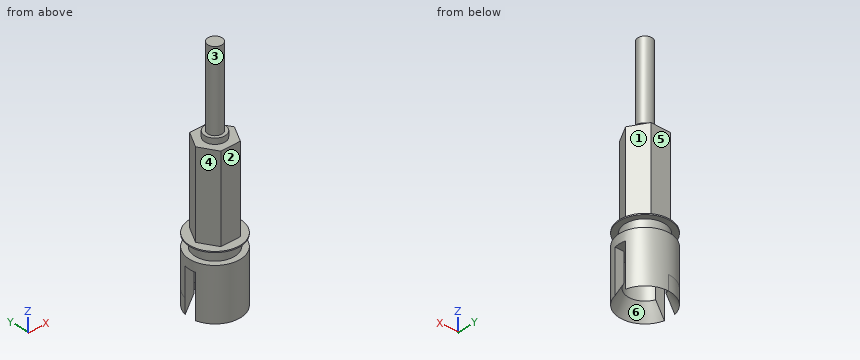
Autodesk Inventor part; units mm, degrees
ref_plane "YZ Plane" through (0, 0, 0) normal (1, 0, 0) x (0, 1, 0)
ref_plane "XZ Plane" through (0, 0, 0) normal (0, 1, 0) x (-1, 0, 0)
ref_plane "XY Plane" through (0, 0, 0) normal (0, 0, 1) x (1, 0, 0)
sketch "Sketch1" plane through (0, 0, 0) normal (0, 0, 1) x (1, 0, 0)
  line L0 (2.1997, -3.81) -> (-2.1997, -3.81)
  line L1 (-2.1997, -3.81) -> (-4.3994, 0)
  line L2 (-4.3994, 0) -> (-2.1997, 3.81)
  line L3 (-2.1997, 3.81) -> (2.1997, 3.81)
  line L4 (2.1997, 3.81) -> (4.3994, 0)
  line L5 (4.3994, 0) -> (2.1997, -3.81)
  point P0 (0, 0)
  point P1 (0, 0)
  dimension "d0" = 7.62
extrude "Extrusion1" add sketch "Sketch1" along normal blind 19.05
sketch "Sketch2" plane through (0, 0, 19.05) normal (0, 0, 1) x (1, 0, 0)
  circle A0 centre (0, 0) radius 2.286
  dimension "d3" = 4.572
extrude "Extrusion2" add sketch "Sketch2" along normal blind 1.27
sketch "Sketch3" plane through (0, 0, 20.32) normal (0, 0, 1) x (1, 0, 0)
  circle A0 centre (0, 0) radius 2.286
  circle A1 centre (0, 0) radius 1.5875
  dimension "d6" = 3.175
extrude "Extrusion3" add sketch "Sketch3" along normal blind 17.78 contours A1
thread "Thread1"
sketch "Sketch4" plane through (0, 0, 0) normal (0, 0, -1) x (-1, 0, 0)
  circle A0 centre (0, 0) radius 5.715
  dimension "d11" = 11.43
extrude "Extrusion4" add sketch "Sketch4" along normal blind 0.254
sketch "Sketch5" plane through (0, 0, -0.254) normal (0, 0, -1) x (-1, 0, 0)
  circle A0 centre (0, 0) radius 5.715
  circle A1 centre (0, 0) radius 4.445
  dimension "d14" = 8.89
extrude "Extrusion5" add sketch "Sketch5" along normal blind 2.54 contours A1
sketch "Sketch6" plane through (0, 0, -2.794) normal (0, 0, -1) x (-1, 0, 0)
  circle A0 centre (0, 0) radius 4.445
  circle A1 centre (0, 0) radius 5.715
  dimension "d17" = 11.43
extrude "Extrusion6" add sketch "Sketch6" along normal blind 2.032 contours A0 | A1
sketch "Sketch7" plane through (0, 0, -4.826) normal (0, 0, -1) x (-1, 0, 0)
  circle A0 centre (0, 0) radius 5.715
  circle A1 centre (0, 0) radius 5.715
  line L0 (0, 6.5237) -> (0, -6.5237) construction
  arc A2 (-3.5921, -1.27) -> (3.5921, -1.27) centre (0, 0) ccw
  arc A3 (3.5921, 1.27) -> (-3.5921, 1.27) centre (0, 0) ccw
  arc A4 (-5.5721, -1.27) -> (5.5721, -1.27) centre (0, 0) ccw
  arc A5 (5.5721, 1.27) -> (-5.5721, 1.27) centre (0, 0) ccw
  arc A6 (-3.5921, 1.27) -> (-3.5921, -1.27) centre (0, 0) ccw
  arc A7 (-5.5721, 1.27) -> (-5.5721, -1.27) centre (0, 0) ccw
  arc A8 (3.5921, -1.27) -> (3.5921, 1.27) centre (0, 0) ccw
  arc A9 (5.5721, -1.27) -> (5.5721, 1.27) centre (0, 0) ccw
  point P0 (-5.715, 1.27)
  point P1 (-5.715, -1.27)
  point P2 (5.715, 1.27)
  point P3 (5.715, -1.27)
extrude "Extrusion8" add sketch "Sketch7" along normal blind 6.35
sketch "Sketch13" plane through (0, 0, 0) normal (1, 0, 0) x (0, 1, 0)
  line L0 (2.286, 20.32) -> (2.286, 19.05)
  line L1 (2.286, 19.05) -> (3.81, 19.05)
  line L2 (3.81, 19.05) -> (3.81, 0)
  line L3 (3.81, 0) -> (5.715, 0)
  line L4 (5.715, 0) -> (5.715, -0.254)
  line L5 (5.715, -0.254) -> (4.445, -0.254)
  line L6 (4.445, -0.254) -> (4.445, -2.794)
  line L7 (4.445, -2.794) -> (5.715, -2.794)
  line L8 (5.715, -2.794) -> (5.715, -11.176)
  line L9 (5.715, -11.176) -> (3.81, -11.176)
  line L10 (3.81, -11.176) -> (3.81, -4.826)
  line L11 (3.81, -4.826) -> (-3.81, -4.826)
  line L12 (-3.81, -4.826) -> (-3.81, -11.176)
  line L13 (-3.81, -11.176) -> (-5.715, -11.176)
  line L14 (-5.715, -11.176) -> (-5.715, -2.794)
  line L15 (-5.715, -2.794) -> (-4.445, -2.794)
  line L16 (-4.445, -2.794) -> (-4.445, -0.254)
  line L17 (-4.445, -0.254) -> (-5.715, -0.254)
  line L18 (-5.715, -0.254) -> (-5.715, 0)
  line L19 (-5.715, 0) -> (-3.81, 0)
  line L20 (-3.81, 0) -> (-3.81, 19.05)
  line L21 (-3.81, 19.05) -> (-2.286, 19.05)
  line L22 (-2.286, 19.05) -> (-2.286, 20.32)
  line L23 (-2.286, 20.32) -> (-1.5875, 20.32)
  line L24 (-1.5875, 20.32) -> (-1.5875, 38.1)
  line L25 (-1.5875, 38.1) -> (1.5875, 38.1)
  line L26 (1.5875, 38.1) -> (1.5875, 20.32)
  line L27 (1.5875, 20.32) -> (2.286, 20.32)
  line L28 (5.715, -11.176) -> (5.715, -14.4756)
  line L29 (5.715, -14.4756) -> (3.81, -11.176)
  line L30 (3.81, -11.176) -> (5.715, -11.176)
  line L31 (0, -24.9907) -> (0, 48.6151)
  point P0 (0, 0)
  dimension "d32" = 30
revolve "Revolution1" add sketch "Sketch13" angle 360 about axis through (0, 0, -10) along (0, 0, 1) contours L9 L28 L29
sketch "Sketch16" plane through (0, 0, -4.826) normal (0, 0, -1) x (-1, 0, 0)
  circle A0 centre (0, 0) radius 3.81
  line L0 (-5.5721, 1.27) -> (-3.5921, 1.27)
  line L1 (-3.5921, -1.27) -> (-5.5721, -1.27)
  arc A1 (-3.5921, 1.27) -> (-3.5921, -1.27) centre (0, 0) ccw
  arc A2 (-5.5721, 1.27) -> (-5.5721, -1.27) centre (0, 0) ccw
  circle A3 centre (0, 0) radius 5.715
  line L2 (5.5721, -1.27) -> (3.5921, -1.27)
  line L3 (3.5921, 1.27) -> (5.5721, 1.27)
  arc A4 (3.5921, -1.27) -> (3.5921, 1.27) centre (0, 0) ccw
  arc A5 (5.5721, -1.27) -> (5.5721, 1.27) centre (0, 0) ccw
  dimension "d47" = 360
extrude "Extrusion9" cut sketch "Sketch16" along normal up to surface contours A0 L3 A3 L2 | A0 L1 A2 L0
properties part number "Shaft"
Could you check a few things on this model? Use its own coordinates, in mm. Face numbers are marked on the shaded views. A direction names the side the tool comes from. Round coordinates to 2 decimals unless told otherwise and drop trailing zeros. Loops run counter-clockwise (first coordinate to the right, second up) from the corner with the lowest first, then second, coordinate; pieces in that order, holes last. Notation, with made-up numbers: M 3.25,50 L 8.25,50 A17 cw 8.25,71 Z; hole C 65.25,1.25 d3. An arc over 180 degrees is marked long. Write item = value, one per line.
1. I want a section at A-A, the plane z = -10. Write out the boundary of the cut face in (x, y) (3 decimals), and give its area (3 significant figures).
Results below:
outline = M -5.572,-1.27 A5.715 ccw 5.572,-1.27 L 3.592,-1.27 A3.81 cw -3.592,-1.27 Z; M -5.572,1.27 L -3.592,1.27 A3.81 cw 3.592,1.27 L 5.572,1.27 A5.715 ccw Z
area = 47.2 mm²
2. I want a section at B-B, the plane z = 9. Write out the boundary of the cut face in (x, y).
Results below:
outline = M -4.4,0 L -2.2,-3.81 L 2.2,-3.81 L 4.4,0 L 2.2,3.81 L -2.2,3.81 Z
3. I want a section at D-D, the plane z = -1. Write out the boundary of the cut face in (x, y) (3 decimals).
Results below:
outline = C 0,0 d8.89
4. Will these pins go through, and if not, where does the flat tip stop? P1, Ø2, axis at x = 3.5, y = 4, coming from the +Z side; P2, Ø4, axis at x = 0.5, y = 0.5, coming from the -Z side; P3, Ø6, axis at x = 0.5, y = 2.5, coming from the -Z side.
Results below:
P1 = 0
P2 = -4.83
P3 = -14.19
5. Which directions (+Z, -Z, +X, -X, +Y, -Y) give clear straight access to the entire face, cutting with the end or side of a thin tool? Please do the marked faces 1 and 2.
Results below:
face_1 = +Z, +X, +Y
face_2 = +Z, +X, -X, -Y
6. I need wall thicknesses on probe 1 along Z at (x, y) = (1.25, -1.5); probe 2 along Z at (x, y) = (-5, -0.5); probe 3 along Z at (x, y) = (-3, -1.5). Which ranges of each line are inside material? Lowest first, please.
Results below:
probe_1 = -4.83 to 20.32
probe_2 = -4.83 to -2.79, -0.25 to 0
probe_3 = -4.83 to 19.05
7. Thinking about a two-plate mould opening in Y: for the marked faces 3, 4, 5 and 6, which applies, +Y half, -Y half, draft (parallel to the pull), parting line (faces both ways), or undercut?
Results below:
face_3 = parting line
face_4 = -Y half
face_5 = +Y half
face_6 = undercut
8. I want a section at C-C, the plane z = 21.5. Write out the boundary of the cut face in (x, y) (1 decimal).
Results below:
outline = C 0,0 d3.2
